The listing builds one solid part. Answer for the finished solid, in the listing's coordinates (mm). Face numbers are marked on the shaded views. A direction names the side the tool comes from. Coordinates: 2 decimals unless noted, no trailing zeros. Write each loop counter-clockwise with the first axis right and the second up, starting at its lowest first coordinate (ties: lowest second). Pieces come first, ordered by that corner, then holes. Notation, with made-up numbers: M 36,38.25 L 94,38.25 A8 ccw 94,46.25 Z; hole C 26,88 d7. An arc over 180 degrees is marked long. Answer as CSV lines item,"result". Start each with the question number.
Autodesk Inventor part; units mm, degrees
ref_plane "YZ Plane" through (0, 0, 0) normal (1, 0, 0) x (0, 1, 0)
ref_plane "XZ Plane" through (0, 0, 0) normal (0, 1, 0) x (-1, 0, 0)
ref_plane "XY Plane" through (0, 0, 0) normal (0, 0, 1) x (1, 0, 0)
sketch "Sketch1" plane through (0, 0, 0) normal (0, 1, 0) x (-1, 0, 0)
  line L0 (0, 0) -> (53.975, 0)
  line L1 (53.975, 0) -> (53.975, -127)
  line L2 (53.975, -127) -> (0, -127)
  line L3 (0, -127) -> (0, 0)
  dimension "d0" = 53.975
  dimension "d1" = 127
extrude "Extrusion1" add sketch "Sketch1" along normal blind 3.175
sketch "Sketch2" plane through (0, 3.175, 0) normal (0, 1, 0) x (1, 0, 0)
  line L0 (0, 127) -> (-53.975, 127)
  line L1 (0, 0) -> (-3.175, 0)
  line L2 (-3.175, 0) -> (-3.175, 127)
  line L3 (-3.175, 127) -> (0, 127)
  line L4 (0, 127) -> (0, 0)
  dimension "d4" = 3.175
extrude "Extrusion2" add sketch "Sketch2" along normal blind 25.4
sketch "Sketch3" plane through (-3.175, 3.175, -127) normal (-1, 0, 0) x (0, 0, 1)
  circle A0 centre (63.5, 12.7) radius 6.35
  line L0 (0, 25.4) -> (127, 25.4)
  line L1 (0, 0) -> (0, 25.4)
  point P0 (127, -3.175)
  dimension "d7" = 12.7
  dimension "d8" = 12.7
  dimension "d9" = 63.5
extrude "Extrusion3" cut sketch "Sketch3" against normal blind 3.175
properties part number "First Pivot Point"
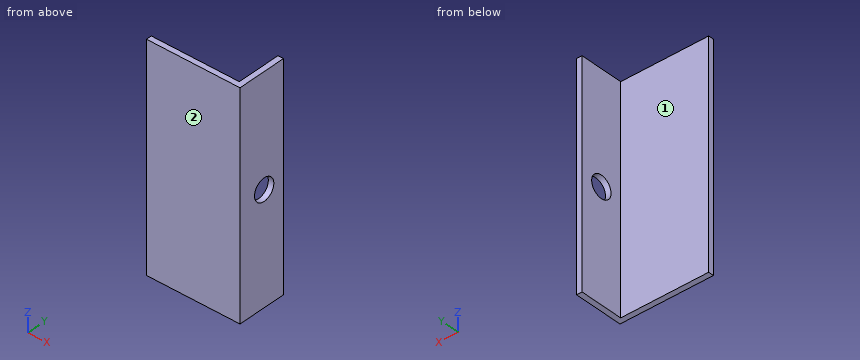
1) The part is cut by section B-B (z = -63.5). Determine the outline of the cut face in (x, y) (3 decimals), then the cut area to 3 significant figures.
2) Which of the six approach directions +Z, -Z, +X, -X, +Y, -Y give full straight-line access (tool end or side, diameter ignored) to the marked faces 1 and 2?
3) The part is cut by section A-A (y = 18). Determine the outline of the cut face in (x, z) (3 decimals).
4) Find the intervals of material crossed by line 1 (Y direction, x = -0.75, z = -63.5) (3 decimals); line 2 (X direction, y = 5.5, z = -90) (3 decimals); line 3 (Y direction, x = -25.5, z = -68) (3 decimals), in increasing order. Write a range as from..to.
5) Each of these flat-tipped pins is pushed along its axis until it touches: P1, Ø15, axis at x = -19.5, z = -86, coming from the +Y side (3 decimals); P2, Ø12, axis at y = 24.5, z = -109, coming from the -X side (3 decimals). Where does it stop, or does it pass through?
6) The part is cut by section D-D (y = 7.25). Determine the outline of the cut face in (x, z) (3 decimals), then the cut area to 3 significant figures.
7) The part is cut by section C-C (z = -111). Determine the outline of the cut face in (x, y) (3 decimals).
Completed:
1,outline,"M -53.975,0 L 0,0 L 0,9.525 L -3.175,9.525 L -3.175,3.175 L -53.975,3.175 Z; M -3.175,22.225 L 0,22.225 L 0,28.575 L -3.175,28.575 Z"
1,area,"212 mm²"
2,face 1,"+Z, -Z, -X, +Y"
2,face 2,"+Z, -Z, +X, -X, -Y"
3,outline,"M -3.175,-127 L 0,-127 L 0,-69.484 L -3.175,-69.484 Z; M -3.175,-57.516 L 0,-57.516 L 0,0 L -3.175,0 Z"
4,line 1,"0..9.525, 22.225..28.575"
4,line 2,"-3.175..0"
4,line 3,"0..3.175"
5,P1,"y = 3.175"
5,P2,"x = -3.175"
6,outline,"M -3.175,-127 L 0,-127 L 0,0 L -3.175,0 Z"
6,area,"403 mm²"
7,outline,"M -53.975,0 L 0,0 L 0,28.575 L -3.175,28.575 L -3.175,3.175 L -53.975,3.175 Z"
